Source: three-view drawing plus pictorial views. Frame: mm from the lowest corner of the part. Round coordinates to 2 decimals unless told otherwise and drop trailing zeros. Write each loop counter-clockwise with the first axis right and the second up, starting at its lowest first coordinate (ties: lowest second). Pieces come first, ordered by that corner, then holes. Notation, with made-up numbers: (31, 56) -> (79, 56) arc R18 cw to (79, 90) -> close; hole circle Ø11 at (23.25, -35). An arc over 180 degrees is marked (long way). Put each result on its own line as item: value.
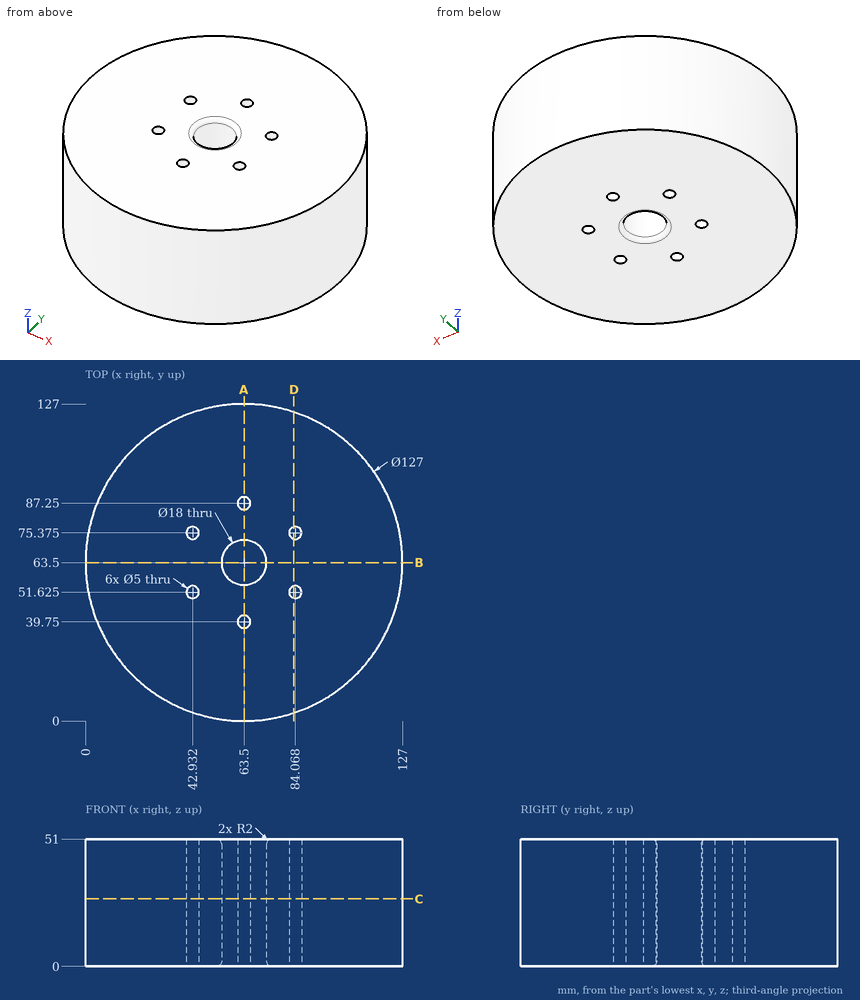
Q1. Cut plane A-A on x = 63.5. Output: boundary loops of the cut face in (y, z), and give its area (3 significant figures).
Ans:
outline: (0, 0) -> (37.25, 0) -> (37.25, 51) -> (0, 51) -> close; (42.25, 0) -> (52.5, 0) arc R2 ccw to (54.5, 2) -> (54.5, 49) arc R2 ccw to (52.5, 51) -> (42.25, 51) -> close; (72.5, 2) arc R2 ccw to (74.5, 0) -> (84.75, 0) -> (84.75, 51) -> (74.5, 51) arc R2 ccw to (72.5, 49) -> close; (89.75, 0) -> (127, 0) -> (127, 51) -> (89.75, 51) -> close
area: 5,050 mm^2
Q2. Pin query (flat end, axial travel): pin 1 (4 mm diameter, centred on y = 102.5, z = 25.5, fed in from +X); pin 2 (20.5 mm diameter, centred on x = 63.5, y = 63.5, fed in from +Z); pin 3 (5 mm diameter, centred on x = 61, z = 27.5, fed in from -Y); pin 4 (4.5 mm diameter, centred on x = 84.07, y = 51.62, fed in from -Z). Return the tip coordinate at first contact, or that it passes through.
Ans:
pin 1: stops at x = 115.11
pin 2: stops at z = 50.85
pin 3: stops at y = 0
pin 4: passes through
Q3. Cut plane B-B on y = 63.5. Output: boundary loops of the cut face in (x, z), and give its area (3 significant figures).
Ans:
outline: (0, 0) -> (52.5, 0) arc R2 ccw to (54.5, 2) -> (54.5, 49) arc R2 ccw to (52.5, 51) -> (0, 51) -> close; (72.5, 2) arc R2 ccw to (74.5, 0) -> (127, 0) -> (127, 51) -> (74.5, 51) arc R2 ccw to (72.5, 49) -> close
area: 5,560 mm^2
Q4. Material intervals for line 1 (Y direction, x = 63.5, z = 39); line 2 (X direction, y = 63, z = 18); line 3 (X direction, y = 74.5, z = 27.5), sorted ascending. Write a range as [from, to].
Ans:
line 1: y = [0, 37.25], [42.25, 54.5], [72.5, 84.75], [89.75, 127]
line 2: x = [0, 54.51], [72.49, 127]
line 3: x = [0.96, 40.59], [45.27, 81.73], [86.41, 126.04]
Q5. Cut plane C-C on z = 27. Output: boundary loops of the cut face in (x, y) (3 decimals), and give its area (3 significant figures).
Ans:
outline: circle Ø127 at (63.5, 63.5); hole circle Ø5 at (42.932, 51.625); hole circle Ø5 at (42.932, 75.375); hole circle Ø18 at (63.5, 63.5); hole circle Ø5 at (63.5, 39.75); hole circle Ø5 at (63.5, 87.25); hole circle Ø5 at (84.068, 51.625); hole circle Ø5 at (84.068, 75.375)
area: 12,300 mm^2
Q6. Cut plane D-D on x = 83.5. Output: boundary loops of the cut face in (y, z), and give its area (3 significant figures).
Ans:
outline: (3.23, 0) -> (49.19, 0) -> (49.19, 51) -> (3.23, 51) -> close; (54.06, 0) -> (72.94, 0) -> (72.94, 51) -> (54.06, 51) -> close; (77.81, 0) -> (123.77, 0) -> (123.77, 51) -> (77.81, 51) -> close
area: 5,650 mm^2
